Autodesk Inventor part; units mm, degrees
ref_plane "Work Plane1" through (1.5, 0, 0) normal (1, 0, 0) x (0, 1, 0)
ref_plane "XZ Plane" through (0, 0, 0) normal (0, 1, 0) x (-1, 0, 0)
ref_plane "XY Plane" through (0, 0, 0) normal (0, 0, 1) x (1, 0, 0)
sketch "Sketch1" plane through (0, 0, 0) normal (0, 0, 1) x (1, 0, 0)
  circle A0 centre (0, 0) radius 1.5
  dimension "d0" = 3
extrude "Extrusion1" add sketch "Sketch1" against normal blind 117
ref_plane "Work Plane1" through (1.5, 0, 0) normal (1, 0, 0) x (0, 1, 0)
sketch "Sketch2" plane through (1.5, 0, 0) normal (1, 0, 0) x (0, 1, 0)
  line L0 (1.5, 0) -> (1.5, -117)
  line L1 (1.5, 0) -> (-1.5, 0)
  line L2 (-1.5, 0) -> (-1.5, -117)
  line L3 (1.5, -16) -> (-1.5, -16)
  line L4 (1.5, -66) -> (-1.5, -66)
  line L5 (-1.5, -66) -> (1.5, -66)
  point P0 (0, 0)
  dimension "d4" = 0
  dimension "d5" = 16
  dimension "d6" = 50
  dimension "d17" = 0
  dimension "d18" = 0
  dimension "d19" = 3
  dimension "d20" = 3
bend part "Bend Part1" radius 5 angle 7.5 line through (1.5, -1.5, -66) along (0, 1, 0) centre toward (1, 0, 0) moving side (0, 0, -1) both sides no
sketch "Sketch3" plane through (1.5, 0, 0) normal (1, 0, 0) x (0, 1, 0)
  line L0 (-1.5, -66) -> (1.5, -66)
  line L1 (1.5, -66) -> (-1.5, -66)
  line L2 (-1.5, -66) -> (-1.5, -66.8484)
  line L3 (2.4329, -66) -> (-2.7481, -66)
  line L4 (2.4329, -16) -> (-2.7481, -16)
  point P0 (0, 0)
  dimension "d9" = 50
  dimension "d12" = 50
  dimension "d13" = 3.9329
  dimension "d14" = 3.9329
  dimension "d15" = 1.2481
  dimension "d16" = 1.2481
bend part "Bend Part2" radius 5 angle 7.5 line through (1.5, 2.4329, -16) along (0, -1, 0) centre toward (-1, 0, 0) moving side (0, 0, 1) both sides no
thread "Thread1"
properties part number "32 - Eccentric Disk Rod" material "Steel AISI 1020 107 HR"
Geometry: final body of the model. Coordinates: model frame, mm. A direction names the side the tool comes from. Coordinates: 2 decimals unless noted, no trailing zeros. Loops run counter-clockwise (first coordinate to the right, second up) from the corner with the lowest first, then second, coordinate; pieces in that order, holes last. Notation, with made-up numbers: M -24,49 L -5,49 A11 ccw -5,53 Z; hole C 22,-0.75 d10. An arc over 180 degrees is marked long. One line per item, written item: value. Start each with the question number.
1) Reachability of faces 1 (the flat face through (-2.05, 0.02, -0.33)), 2 (the cylindrical face through (-1.5, 0.07, -40.65)) from +Z, -Z, +X, -X, +Y, -Y: full face, straight path, thin tool, end or side. Return the list, or none.
2) Material intervals for L1, parallel to X at y = -0.25, z = -51.5; L2, parallel to Y at x = 4.75, z = -99.5, sorted ascending. Write a range as from..to.
3) Pin query (flat end, axial travel): P1, Ø1.5, axis at x = 7, y = 0.5, coming from the -Z side; P2, Ø3, axis at x = 1.5, z = -30.5, coming from the -Y side; P3, Ø1, axis at y = -1, z = -56, coming from the +X side; P4, Ø1.5, axis at x = -2, z = -81.5, coming from the +Y side. Return the tip coordinate at first contact, or that it passes through.
4) Cut plane A-A (y = 0). Return loops of the section in (x, z), then the cut area to 3 significant figures.
Evaluation:
1. face 1: +Z, -X, +Y, -Y
1. face 2: none
2. L1: -1.48..1.48
2. L2: -1.45..1.45
3. P1: z = -116.81
3. P2: y = -1.5
3. P3: x = 1.41
3. P4: through
4. outline: M -3.52,-0.52 L -1.52,-15.74 A2 cw -1.5,-16 L -1.5,-66 A8 ccw -1.43,-67.04 L 5.14,-116.96 L 8.11,-116.57 L 1.54,-66.65 A5 cw 1.5,-66 L 1.5,-16 A5 ccw 1.46,-15.35 L -0.55,-0.13 Z
4. area: 351 mm^2
